from build123d import *

# Parameters (mm, degrees)
SKETCH1_R           = 30
BOSS_EXTRUDE1_DEPTH = 25
CHAMFER1_SIZE       = 5


with BuildPart() as part:
    # Sketch1 → Boss-Extrude1 (new body)
    with BuildSketch(Plane.XY):
        with BuildLine():
            Line((1440, -50), (-1440, -50))
            ThreePointArc((-1440, -50), (-1490, 0), (-1440, 50))
            Line((-1440, 50), (1440, 50))
            ThreePointArc((1440, 50), (1490, 0), (1440, -50))
        make_face()
        with Locations((-1440, 0)):
            Circle(SKETCH1_R, mode=Mode.SUBTRACT)
        with Locations(Location((1440, 0, 0), (0, 0, 180))):
            Circle(SKETCH1_R, mode=Mode.SUBTRACT)
        with Locations((-115, 0)):
            Circle(SKETCH1_R, mode=Mode.SUBTRACT)
    extrude(amount=BOSS_EXTRUDE1_DEPTH)

    # Chamfer1
    chamfer1_edges = [part.edges().sort_by_distance(p)[0] for p in [
        (1490, 0, 25),
        (-1470, 0, 0),
        (-1470, 0, 25),
        (0, 50, 25),
        (1470, 0, 0),
        (1470, 0, 25),
        (-145, 0, 0),
        (-145, 0, 25),
        (-1490, 0, 25),
        (0, 50, 0),
        (1490, 0, 0),
        (0, -50, 0),
        (-1490, 0, 0),
        (0, -50, 25),
    ]]
    chamfer(chamfer1_edges, length=CHAMFER1_SIZE)


solid = part.part
Model file for the job. Use its own axes, mm. Round coordinates to 2 decimals unless told otherwise and drop trailing zeros. Loops run counter-clockwise (first coordinate to the right, second up) from the corner with the lowest first, then second, coordinate; pieces in that order, holes last. Notation, with made-up numbers: (-39.5, 26) -> (-7.5, 26) arc R13 ccw to (-7.5, 48) -> close; hole circle Ø6 at (-32, 41.5). An arc over 180 degrees is marked (long way). Answer as CSV lines item,"result". Start each with the question number.
1) Slice it at A-A (x = -115). List the corners of the cut face in (y, z), plus the area to 3 significant figures.
2) Slice it at B-B (y = 0). State how many separate pieces and enclosed holes the cut face has, plus the area to 3 significant figures.
3) Mould opens along X. For faces 1 (the face through (21, 1, 25)), 2 (the face through (-1485.23, -0.99, 0.24)), 3 (the face through (-1412, -11.61, 20.31)) say: +X half, -X half, draft (parallel to the pull), parting line (faces both ways), or undercut.
4) Pin check, flat tips, straight feed: P1, Ø3, axis at y = -24, z = 11, coming from the +X side; P2, Ø4, axis at y = 39.5, z = 14, coming from the -X side; P3, Ø8, axis at y = 10.5, z = 5, coming from the +X side. Stop position of each tip, or through.
5) Probe line 1 along Y through (x, z) = (-1440, 10.5); line 2 along X through (y, z) = (-26, 2.75); line 3 along X through (y, z) = (18, 22.25). List the from-to ranges inside material, lowest first.
Filled in:
1,outline,"(-50, 5) -> (-45, 0) -> (-35, 0) -> (-30, 5) -> (-30, 20) -> (-35, 25) -> (-45, 25) -> (-50, 20) -> close; (30, 5) -> (35, 0) -> (45, 0) -> (50, 5) -> (50, 20) -> (45, 25) -> (35, 25) -> (30, 20) -> close"
1,area,"900 mm2"
2,separate pieces,"4"
2,enclosed holes,"0"
2,area,"69,800 mm2"
3,face 1,"draft"
3,face 2,"-X half"
3,face 3,"undercut"
4,P1,"stops at x = 1484.65"
4,P2,"stops at x = -1473.07"
4,P3,"stops at x = 1489.58"
5,line 1,"y = -50 to -30, 30 to 50"
5,line 2,"x = -1480.05 to -1459.08, -1420.92 to -134.08, -95.92 to 1420.92, 1459.08 to 1480.05"
5,line 3,"x = -1484.23 to -1466.76, -1413.24 to -141.76, -88.24 to 1413.24, 1466.76 to 1484.23"
